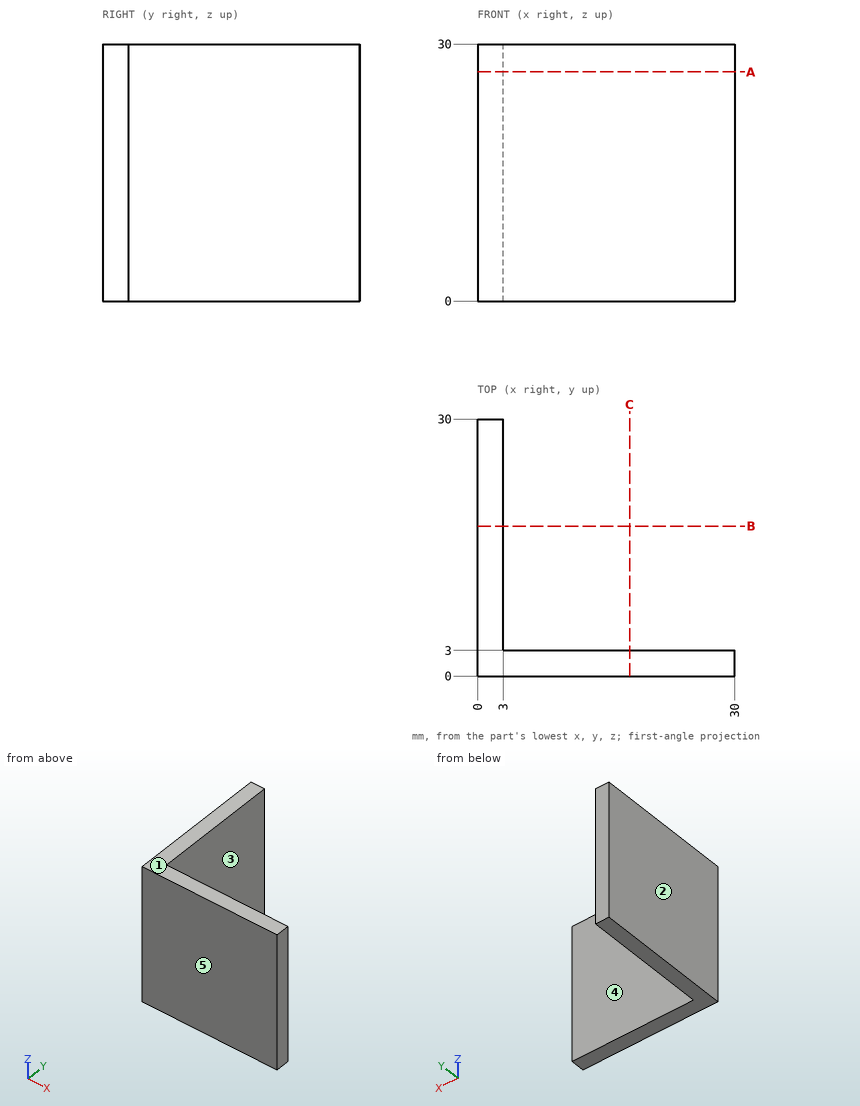
Print and shaded views of the part. All mm, measured from the part's lowest x, y and z. A direction names the side the tool comes from. Coordinates: 2 decimals unless noted, no trailing zeros. Loops run counter-clockwise (first coordinate to the right, second up) from the corner with the lowest first, then second, coordinate; pieces in that order, holes last. Notation, with made-up numbers: (65, 67.5) - (119, 67.5) arc R30 cw to (119, 90.5) - close; hole circle Ø10 at (-32, -29). An arc over 180 degrees is marked (long way). Use one line per item in the form item = value. Start each with the question number.
1) Drill centre line: L1, parallel to X at y = 9.75, z = 2. Where is it in solid material? Low to high. Write a range as from..to.
2) Tool access for the marked faces 4 and 5: list every direction of +Z, -Z, +X, -X, +Y, -Y with a clear straight run to the whole face (end or side of a thin tool).
3) Band-saw the part on B-B (y = 17.5). Give the cut face in (x, z).
4) Two-plate mould, pull along X, no slides. Class the marked faces 1, 2 and 3: +X half, -X half, draft (parallel to the pull), parting line (faces both ways), or undercut.
5) Band-saw the part on A-A (z = 26.75). Give the cut face in (x, y), and give its area (3 significant figures).
6) Flat gauge pins, fed straight in: pin 1 (12 mm diameter, centred on y = 8, z = 12.5, fed in from +X); pin 2 (12 mm diameter, centred on y = 19, z = 12.5, fed in from +X). Where does each tip first touch, or does it go through?
Check values:
q1.L1 = 0..3
q2.face_4 = +Z, -Z, +X, +Y
q2.face_5 = +Z, -Z, +X, -X, -Y
q3.outline = (0, 0) - (3, 0) - (3, 30) - (0, 30) - close
q4.face_1 = draft
q4.face_2 = -X half
q4.face_3 = +X half
q5.outline = (0, 0) - (30, 0) - (30, 3) - (3, 3) - (3, 30) - (0, 30) - close
q5.area = 171 mm2
q6.pin_1 = 30
q6.pin_2 = 3
